The model under review builds one solid part; all positions refer to its coordinate system, in mm. Face numbers are marked on the shaded views. A direction names the side the tool comes from. Round coordinates to 2 decimals unless told otherwise and drop trailing zeros. Order: outer loops, then holes, each group sorted by start corner. A loop starts at its lowest first (then second) coordinate and runs counter-clockwise, first axis right, second up. Notation, with made-up numbers: M 29.25,-9.75 L 71.25,-9.75 A27 ccw 71.25,22.25 Z; hole C 66.25,-11 d3. An arc over 180 degrees is marked long. Answer as a JSON object with one key per item and string values. Group by question number.
1) To check wall thickness, follow line 1 (Y direction, x = 1.8, z = 0.5); line 2 (Y direction, x = 1.7, z = -2.25); line 3 (X direction, y = -0.5, z = 0.5). State the ranges of each line that lie inside material, in increasing order.
2) Insertion check: pin 1 Ø3 at (y, z) = (-9.5, -1.5) entering from +X; pin 2 Ø2 at (y, z) = (-13, 0.5) entering from -X. Each pin has a flat end and moves straight along its axis. Give the tip position at first contact, or say it passes through.
3) Consider section C-C, the plane y = -3. Write out the cut boundary in (x, z).
4) Consider section B-B, the plane x = 0. Write out the cut boundary in (y, z).
5) Consider section A-A, the plane z = 0. Write out the cut boundary in (x, y), then the cut area to 3 significant figures.
6) For the marked faces 1 and 2, list the 3-axis set-ups (+Z, -Z, +X, -X, +Y, -Y) from which the entire face can be reached by the end or side of a thin tool; tool diameter is ignored.
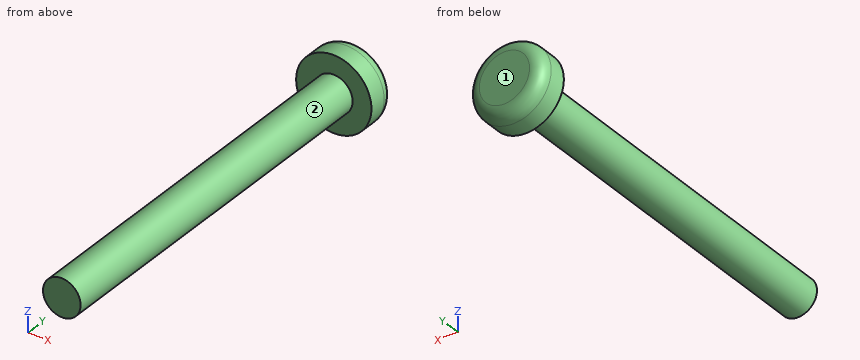
Autodesk Inventor part; units mm, degrees
ref_plane "YZ Plane" through (0, 0, 0) normal (1, 0, 0) x (0, 1, 0)
ref_plane "XZ Plane" through (0, 0, 0) normal (0, 1, 0) x (-1, 0, 0)
ref_plane "XY Plane" through (0, 0, 0) normal (0, 0, 1) x (1, 0, 0)
sketch "Esboço1" plane through (0, 0, 0) normal (0, 1, 0) x (-1, 0, 0)
  circle A0 centre (0, 0) radius 3
  dimension "d0" = 6
extrude "Extrusão1" add sketch "Esboço1" along normal blind 2.4
sketch "Esboço2" plane through (0, 0, 0) normal (0, -1, 0) x (1, 0, 0)
  circle A0 centre (0, 0) radius 1.5
  dimension "d3" = 3
extrude "Extrusão2" add sketch "Esboço2" along normal blind 30
thread "Rosca1"
fillet "Arredondamento1" radius 1 1 edges at (3, 2.4, 0)
properties part number "Parafuso m3x25"
Results list:
{
 "1": {"line 1": "0 to 2.4", "line 2": "0 to 1.97", "line 3": "-1.41 to 1.41"},
 "2": {"pin 1": "x = 1.5", "pin 2": "x = -1.5"},
 "3": {"outline": "C 0,0 d3"},
 "4": {"outline": "M -30,-1.5 L 0,-1.5 L 0,-3 L 1.4,-3 A1 ccw 2.4,-2 L 2.4,2 A1 ccw 1.4,3 L 0,3 L 0,1.5 L -30,1.5 Z"},
 "5": {"outline": "M -3,0 L -1.5,0 L -1.5,-30 L 1.5,-30 L 1.5,0 L 3,0 L 3,1.4 A1 ccw 2,2.4 L -2,2.4 A1 ccw -3,1.4 Z", "area": "104 mm^2"},
 "6": {"face 1": "+Z, -Z, +X, -X, +Y", "face 2": "-Y"}
}
